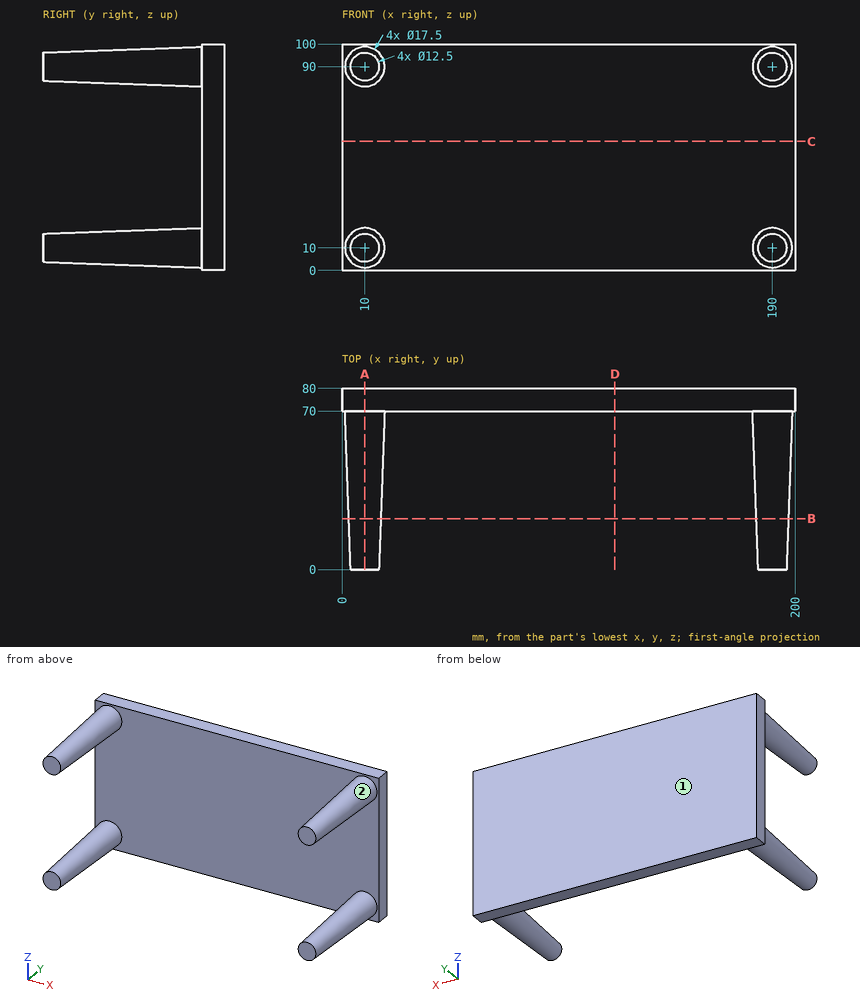
For this review, use the dimensioned drawing (mm, ordinates from the lowest corner) and the shaded views. Round coordinates to 2 decimals unless told otherwise and drop trailing zeros. Loops run counter-clockwise (first coordinate to the right, second up) from the corner with the lowest first, then second, coordinate; pieces in that order, holes last. Notation, with made-up numbers: M -25.5,44.25 L -19.5,44.25 A15 ccw -19.5,48.25 Z; hole C 33.5,55.25 d9. An arc over 180 degrees is marked long. Answer as a JSON object with one key per item and string values.
(1) Take a section at A-A on x = 10. Give the boundary of the cut face in (y, z), and give its area (3 significant figures).
Resolved:
{"outline": "M 0,3.75 L 70,1.25 L 70,0 L 80,0 L 80,100 L 70,100 L 70,98.75 L 0,96.25 L 0,83.75 L 70,81.25 L 70,18.75 L 0,16.25 Z", "area": "3,100 mm²"}
(2) Take a section at C-C on z = 57. Give the boundary of the cut face in (x, y), and give its area (3 significant figures).
Resolved:
{"outline": "M 0,70 L 200,70 L 200,80 L 0,80 Z", "area": "2,000 mm²"}
(3) Draft analysis for pull direction X (two halves, no side actions). For the marked faces 1 and 2, state which applies: released by +X, released by -X, zero draft, split by the parting line, or undercut.
Resolved:
{"face 1": "zero draft", "face 2": "undercut"}
(4) To check wall thickness, follow line 1 along Y through (x, z) = (112.5, 89); line 2 along Z through (x, y) = (187, 43); line 3 along X through (y, z) = (41, 15.5). State the ranges of each line that lie inside material, in increasing order.
Resolved:
{"line 1": "70 to 80", "line 2": "2.82 to 17.18, 82.82 to 97.18", "line 3": "4.59 to 15.41, 184.59 to 195.41"}
(5) Take a section at D-D on x = 120.5. Give the boundary of the cut face in (y, z), and give its area (3 significant figures).
Resolved:
{"outline": "M 70,0 L 80,0 L 80,100 L 70,100 Z", "area": "1,000 mm²"}
(6) Take a section at B-B on y = 22.5. Give the boundary of the cut face in (x, z), and give its area (3 significant figures).
Resolved:
{"outline": "C 10,10 d14.11; C 10,90 d14.11; C 190,10 d14.11; C 190,90 d14.11", "area": "625 mm²"}
